Geometry check sheet. Reference: the model listing, model coordinates, mm. Face numbers are marked on the shaded views. A direction names the side the tool comes from. Round coordinates to 2 decimals unless told otherwise and drop trailing zeros. Loops run counter-clockwise (first coordinate to the right, second up) from the corner with the lowest first, then second, coordinate; pieces in that order, holes last. Notation, with made-up numbers: (-11, -36.5) -> (22, -36.5) arc R17 cw to (22, -18.5) -> close; hole circle Ø1 at (-17.5, 85.25). An arc over 180 degrees is marked (long way). Use a Markdown table: item, result. Add a question column.
Q1. Sectioned sample at C-C, the plane z = 15. Enter the section's corners in (x, y).
Q2. Sectioned sample at A-A, the plane y = 0. Enter the section's corners in (x, z).
Q3. Release check for a two-part mould opening along Y. For the marked faces 3, 4, 5 and 6 record: released by +Y, released by -Y, zero draft, split by the parting line, or undercut.
Q4. Material ranges on L1, parallel to Z at x = 0, y = 3.75; L2, parallel to Y at x = -2.75, z = 14.25; L3, parallel to X at y = 4.3, z = 25, recorded low to high.
Q5. Gauge pin test, flat end, axial feed: P1, Ø5, axis at x = 0, z = 25, coming from the -Y side. Record the tip position at first contact, or that the pin passes through.
Q6. Sectioned sample at B-B, the plane x = 2.5. Enter the section's corners in (y, z), then the cut area to 3 significant figures.
Q7. Sectioned sample at D-D, the plane y = 4. Enter the section's corners in (x, z), then the cut area to 3 significant figures.
Q8. Set-up check for the marked faces 1 and 2: record each of +Z, -Z, +X, -X, +Y, -Y from which the full face is reachable in a straight line by a thin tool's end or side.
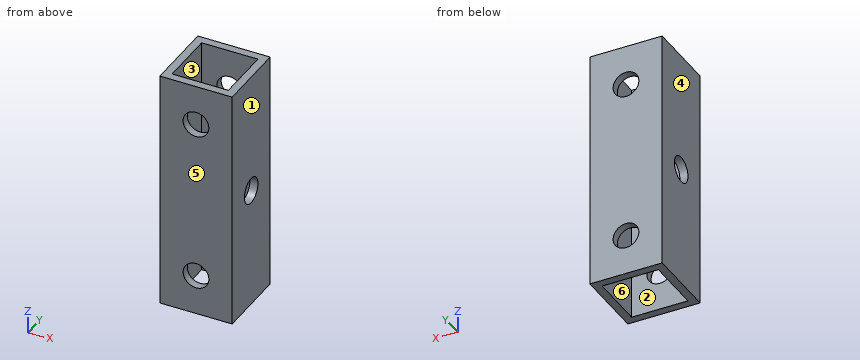
Autodesk Inventor part; units mm, degrees
ref_plane "YZ Plane" through (0, 0, 0) normal (1, 0, 0) x (0, 1, 0)
ref_plane "XZ Plane" through (0, 0, 0) normal (0, 1, 0) x (-1, 0, 0)
ref_plane "XY Plane" through (0, 0, 0) normal (0, 0, 1) x (1, 0, 0)
sketch "スケッチ1" plane through (0, 0, 0) normal (0, 0, 1) x (1, 0, 0)
  line L0 (4.5, -4.5) -> (-4.5, -4.5)
  line L1 (-4.5, -4.5) -> (-4.5, 4.5)
  line L2 (-4.5, 4.5) -> (4.5, 4.5)
  line L3 (4.5, 4.5) -> (4.5, -4.5)
  line L4 (4.5, -4.5) -> (-4.5, 4.5) construction
  line L5 (-4.5, -4.5) -> (4.5, 4.5) construction
  point P0 (0, 0)
  dimension "d0" = 9
  dimension "d1" = 9
extrude "押し出し1" add sketch "スケッチ1" along normal blind 30
shell "シェル1" thickness 1 removed faces 2 at (1.5, -1.5, 0) at (1.5, -1.5, 30)
sketch "スケッチ2" plane through (-4.5, 4.5, 0) normal (0, 1, 0) x (1, 0, 0)
  line L0 (0, 0) -> (9, 0)
  point P0 (4.5, 0)
  point P1 (4.5, -5)
  point P2 (4.5, -25)
  point P3 (4.5, 0)
  dimension "d5" = 20
  dimension "d6" = 5
hole "穴1" at (0, 4.5, 5) at (0, 4.5, 25) direction (0, -1, 0) diameter 3.2 end through all
sketch "スケッチ3" plane through (4.5, -4.5, 0) normal (1, 0, 0) x (0, 0, -1)
  line L0 (0, 9) -> (0, 0)
  line L1 (0, 9) -> (-30, 9)
  line L2 (-30, 0) -> (-30, 9)
  line L3 (0, 0) -> (-30, 0)
  point P0 (0, 4.5)
  point P1 (-15, 4.5)
  point P2 (-15, 9)
  point P3 (0, 4.5)
hole "穴2" at (4.5, 0, 15) direction (-1, 0, 0) diameter 3.2 end through all
properties part number "SqPipeminin"
Values:
| question | item | result |
|---|---|---|
| 1 | outline | (-4.5, -4.5) -> (4.5, -4.5) -> (4.5, -1.6) -> (3.5, -1.6) -> (3.5, -3.5) -> (-3.5, -3.5) -> (-3.5, -1.6) -> (-4.5, -1.6) -> close; (-4.5, 1.6) -> (-3.5, 1.6) -> (-3.5, 3.5) -> (3.5, 3.5) -> (3.5, 1.6) -> (4.5, 1.6) -> (4.5, 4.5) -> (-4.5, 4.5) -> close |
| 2 | outline | (-4.5, 0) -> (-3.5, 0) -> (-3.5, 13.4) -> (-4.5, 13.4) -> close; (-4.5, 16.6) -> (-3.5, 16.6) -> (-3.5, 30) -> (-4.5, 30) -> close; (3.5, 0) -> (4.5, 0) -> (4.5, 13.4) -> (3.5, 13.4) -> close; (3.5, 16.6) -> (4.5, 16.6) -> (4.5, 30) -> (3.5, 30) -> close |
| 3 | face 3 | undercut |
| 3 | face 4 | zero draft |
| 3 | face 5 | released by -Y |
| 3 | face 6 | undercut |
| 4 | L1 | 0 to 3.4, 6.6 to 23.4, 26.6 to 30 |
| 4 | L2 | -4.5 to -3.5, 3.5 to 4.5 |
| 4 | L3 | -4.5 to -1.6, 1.6 to 4.5 |
| 5 | P1 | y = -4.5 |
| 6 | outline | (-4.5, 0) -> (-3.5, 0) -> (-3.5, 30) -> (-4.5, 30) -> close; (3.5, 0) -> (4.5, 0) -> (4.5, 30) -> (3.5, 30) -> close |
| 6 | area | 60.0 mm^2 |
| 7 | outline | (-4.5, 0) -> (4.5, 0) -> (4.5, 30) -> (-4.5, 30) -> close; hole circle Ø3.2 at (0, 5); hole circle Ø3.2 at (0, 25) |
| 7 | area | 254 mm^2 |
| 8 | face 1 | +Z, -Z, +X, +Y, -Y |
| 8 | face 2 | +Z, -Z |
